Input: part model. Units: mm. Frame: model coordinates. Coordinates: 2 decimals unless noted, no trailing zeros. Answer as CSV lines item,"result". Start each with the question number.
Item 1: Material intervals for line 1 along X through (y, z) = (1.1, -155); line 2 along Z through (x, y) = (-42.5, 1); line 3 along Z through (x, y) = (30, 1.2), sorted ascending.
Item 2: Draft query along X for faces 1 (the cylindrical face through (-125.521, 1.014, -173.966)), 2 (the flat face through (-2, 2, -3)). Return one class per face: +X half, -X half, draft (parallel to the pull), parting line (faces both ways), or undercut.
Item 3: First-contact query: pin 1 (2.5 mm diameter, centred on x = 42.5, z = -155, fed in from +Y). Flat tip, straight axial feed; report the tip coordinate or a pass-through.
from build123d import *

# Parameters (mm, degrees)
SKETCH1_W           = 320
SKETCH1_H           = 420
BOSS_EXTRUDE1_DEPTH = 2
SKETCH3_R           = 1.7
SKETCH3_W           = 10
SKETCH3_H           = 15
CUT_EXTRUDE1_DEPTH  = 2
SKETCH5_R           = 4
SKETCH5_R_2         = 8
SKETCH5_W           = 26
SKETCH5_H           = 21.5
CUT_EXTRUDE2_DEPTH  = 2
FILLET1_R           = 5
FILLET2_R           = 2


with BuildPart() as part:
    # Sketch1 → Boss-Extrude1 (new body)
    with BuildSketch(Plane(origin=(0, 0, 0), x_dir=(1, 0, 0), z_dir=(0, 1, 0))):
        Rectangle(SKETCH1_W, SKETCH1_H)
    extrude(amount=BOSS_EXTRUDE1_DEPTH)

    # Sketch3 → Cut-Extrude1 (cut)
    with BuildSketch(Plane(origin=(0, 2, 0), x_dir=(1, 0, 0), z_dir=(0, 1, 0))):
        with Locations((-42.5, 185)):
            Circle(SKETCH3_R)
        with Locations((42.5, 185)):
            Circle(SKETCH3_R)
        with Locations((42.5, 155)):
            Circle(SKETCH3_R)
        with Locations((-42.5, 155)):
            Circle(SKETCH3_R)
        with Locations((27.5, 170)):
            Rectangle(SKETCH3_W, SKETCH3_H)
    extrude(amount=-CUT_EXTRUDE1_DEPTH, mode=Mode.SUBTRACT)

    # Sketch5 → Cut-Extrude2 (cut)
    with BuildSketch(Plane(origin=(0, 2, 0), x_dir=(1, 0, 0), z_dir=(0, 1, 0))):
        with Locations((-125, 170)):
            Circle(SKETCH5_R)
        with Locations((95, 170)):
            Circle(SKETCH5_R_2)
        with Locations((125, 170)):
            Circle(SKETCH5_R)
        with Locations((-90, 170)):
            Rectangle(SKETCH5_W, SKETCH5_H)
    extrude(amount=-CUT_EXTRUDE2_DEPTH, mode=Mode.SUBTRACT)

    # Fillet1
    fillet1_edges = [part.edges().sort_by_distance(p)[0] for p in [
        (160, 1, 210),
        (-160, 1, 210),
        (-160, 1, -210),
        (160, 1, -210),
    ]]
    fillet(fillet1_edges, radius=FILLET1_R)

    # Fillet2
    fillet2_edges = [part.edges().sort_by_distance(p)[0] for p in [
        (32.5, 1, -162.5),
        (22.5, 1, -162.5),
        (22.5, 1, -177.5),
        (32.5, 1, -177.5),
    ]]
    fillet(fillet2_edges, radius=FILLET2_R)


solid = part.part
Determined:
1,line 1,"x = -160 to -44.2, -40.8 to 40.8, 44.2 to 160"
1,line 2,"z = -210 to -186.7, -183.3 to -156.7, -153.3 to 210"
1,line 3,"z = -210 to -177.5, -162.5 to 210"
2,face 1,"undercut"
2,face 2,"draft"
3,pin 1,"passes through"
